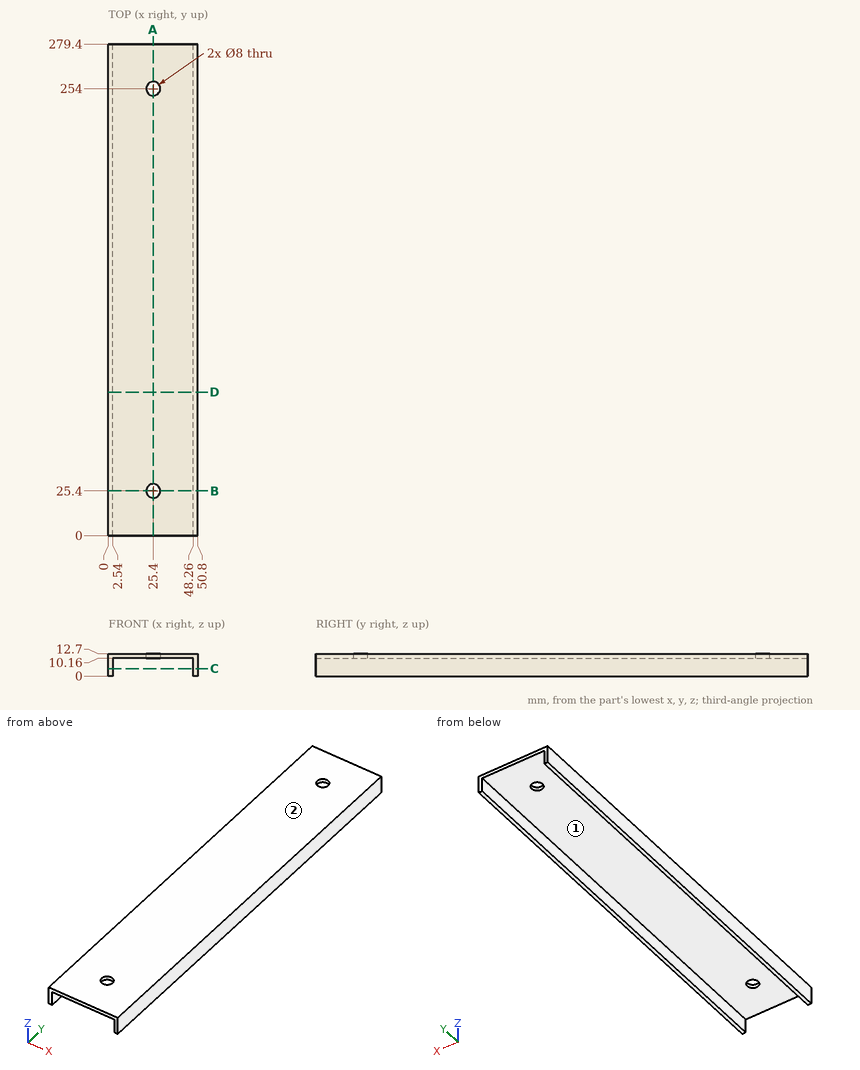
The drawing under review shows one solid part. Ordinate dimensions are in mm from its lowest x, y, z. A direction names the side the tool comes from. Round coordinates to 2 decimals unless told otherwise and drop trailing zeros. Loops run counter-clockwise (first coordinate to the right, second up) from the corner with the lowest first, then second, coordinate; pieces in that order, holes last.
Item 1: Clearance check with a flat-ended pin moving along its axis: pin 1 Ø1.5 at (x, y) = (30, 174.5) entering from -Z. State where the tip first meets the part, or that it passes through.
Determined:
pin 1: stops at z = 10.16
Item 2: For line 1 (Y direction, x = 25.4, z = 10.8); line 2 (X direction, y = 107, z = 1.5); line 3 (Z direction, x = 22, y = 72.5), list the stretches that pass through material, from the lowest coordinate up.
Determined:
line 1: y = 0 to 21.4, 29.4 to 250, 258 to 279.4
line 2: x = 0 to 2.54, 48.26 to 50.8
line 3: z = 10.16 to 12.7
Item 3: Take a section at C-C (z = 4.25). Write out the cut boundary in (x, y).
Determined:
outline: (0, 0) - (2.54, 0) - (2.54, 279.4) - (0, 279.4) - close; (48.26, 0) - (50.8, 0) - (50.8, 279.4) - (48.26, 279.4) - close
Item 4: For the marked faces 1 and 2, list the 3-axis set-ups (+Z, -Z, +X, -X, +Y, -Y) from which the entire face can be reached by the end or side of a thin tool; tool diameter is ignored.
Determined:
face 1: -Z, +Y, -Y
face 2: +Z, +X, -X, +Y, -Y
Item 5: Take a section at D-D (y = 81.5). Write out the cut boundary in (x, z), then the cut area to 3 significant figures.
Determined:
outline: (0, 0) - (2.54, 0) - (2.54, 10.16) - (48.26, 10.16) - (48.26, 0) - (50.8, 0) - (50.8, 12.7) - (0, 12.7) - close
area: 181 mm2
Item 6: Take a section at A-A (x = 25.4). Write out the cut boundary in (y, z).
Determined:
outline: (0, 10.16) - (21.4, 10.16) - (21.4, 12.7) - (0, 12.7) - close; (29.4, 10.16) - (250, 10.16) - (250, 12.7) - (29.4, 12.7) - close; (258, 10.16) - (279.4, 10.16) - (279.4, 12.7) - (258, 12.7) - close
Item 7: Take a section at B-B (y = 25.4). Write out the cut boundary in (x, z).
Determined:
outline: (0, 0) - (2.54, 0) - (2.54, 10.16) - (21.4, 10.16) - (21.4, 12.7) - (0, 12.7) - close; (29.4, 10.16) - (48.26, 10.16) - (48.26, 0) - (50.8, 0) - (50.8, 12.7) - (29.4, 12.7) - close
